Job drawing, mm, ordinate dimensions from the low corner. One solid piece. A direction names the side the tool comes from. Give positions to 0.01 mm unless a question says otherwise; leave off trailing zeros. Write each loop counter-clockwise with the first axis right and the second up, starting at its lowest first coordinate (ties: lowest second). Pieces come first, ordered by that corner, then holes. Notation, with made-up numbers: (81, 70) - (91, 70) arc R19 cw to (91, 104) - close; hole circle Ø8 at (26, 84.5). An arc over 180 degrees is marked (long way). Put each result on its own line as item: value. Start each with the question number.
1. Drop flat-ended pins along their axis: pin 1 (1.8 mm diameter, centred on x = 17.5, z = 3.5, fed in from -Y); pin 2 (1.8 mm diameter, centred on x = 4.5, z = 3.5, fed in from +Y). Give the stop position or say it passes through.
2. Cut at C-C on x = 11.75. List the corners of the cut face in (y, z), and give its area (3 significant figures).
3. Mould opens along Z. For the marked faces 5, 6 and 7 say: +Z half, -Z half, draft (parallel to the pull), parting line (faces both ways), or undercut.
4. Cut at A-A on y = 1.5. List the corners of the cut face in (x, z).
5. Tool access for the marked faces 1, 2, 3 and 4: list every direction of +Z, -Z, +X, -X, +Y, -Y with a clear straight run to the whole face (end or side of a thin tool).
6. Cut at D-D on x = 3.75. List the corners of the cut face in (y, z).
7. Wall check: line 1 (Z direction, x = 3, y = 3.6); line 2 (X direction, y = 3.3, z = 3); line 3 (Y direction, x = 4.25, z = 4.75). Give the ranges that are in metal, low to high.
8. Cut at B-B on z = 4.25. List the corners of the cut face in (x, y).
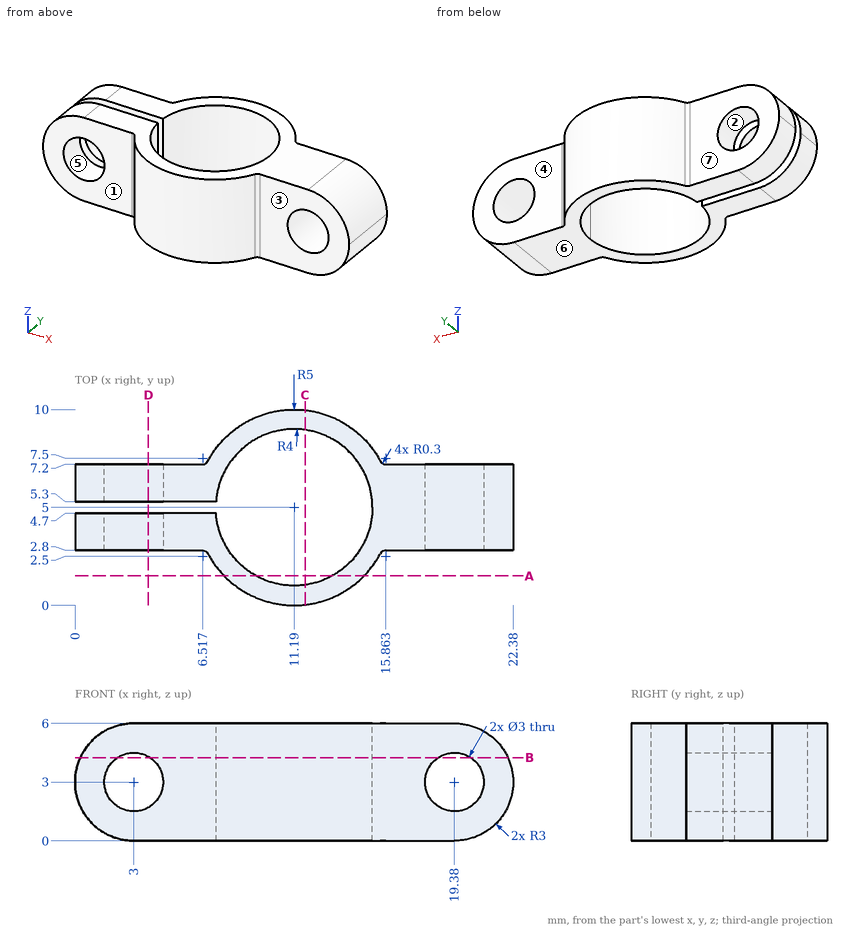
Report:
1. pin 1: stops at y = 2.8
1. pin 2: stops at y = 7.2
2. outline: (0.03, 0) - (1.04, 0) - (1.04, 6) - (0.03, 6) - close; (8.96, 0) - (9.97, 0) - (9.97, 6) - (8.96, 6) - close
2. area: 12.1 mm²
3. face 5: undercut
3. face 6: -Z half
3. face 7: draft
4. outline: (7.62, 0) - (9.25, 0) - (9.25, 6) - (7.62, 6) - close; (13.13, 0) - (14.76, 0) - (14.76, 6) - (13.13, 6) - close
5. face 1: +Z, -Z, -X, -Y
5. face 2: +Y, -Y
5. face 3: +Z, -Z, +X, -Y
5. face 4: +Z, -Z, +X, +Y
6. outline: (2.8, 0) - (4.7, 0) - (4.7, 1.7) - (2.8, 1.7) - close; (2.8, 4.3) - (4.7, 4.3) - (4.7, 6) - (2.8, 6) - close; (5.3, 0) - (7.2, 0) - (7.2, 1.7) - (5.3, 1.7) - close; (5.3, 4.3) - (7.2, 4.3) - (7.2, 6) - (5.3, 6) - close
7. line 1: z = 0 to 1.5, 4.5 to 6
7. line 2: x = 0 to 1.5, 4.5 to 7.57, 14.81 to 17.88, 20.88 to 22.38
7. line 3: y = 2.8 to 4.7, 5.3 to 7.2
8. outline: (0.27, 2.8) - (2.17, 2.8) - (2.17, 4.7) - (0.27, 4.7) - close; (0.27, 5.3) - (2.17, 5.3) - (2.17, 7.2) - (0.27, 7.2) - close; (3.83, 2.8) - (6.52, 2.8) arc R0.3 cw to (6.78, 2.64) arc R5 ccw to (15.6, 2.64) arc R0.3 cw to (15.86, 2.8) - (18.55, 2.8) - (18.55, 7.2) - (15.86, 7.2) arc R0.3 cw to (15.6, 7.36) arc R5 ccw to (6.78, 7.36) arc R0.3 cw to (6.52, 7.2) - (3.83, 7.2) - (3.83, 5.3) - (7.2, 5.3) arc R4 cw (long way) to (7.2, 4.7) - (3.83, 4.7) - close; (20.21, 2.8) - (22.11, 2.8) - (22.11, 7.2) - (20.21, 7.2) - close
